Read the model definition and answer for the solid it produces. Units are mm, in the model's axes. Give positions to 0.01 mm unless a question says otherwise; leave off trailing zeros. Order: outer loops, then holes, each group sorted by start corner. A loop starts at its lowest first (then second) coordinate and runs counter-clockwise, first axis right, second up. Notation, with made-up numbers: M 50.5,14 L 54.5,14 A22 cw 54.5,40 Z; hole C -12,34 d5. An arc over 180 degrees is marked long. One line per item, written item: value.
from build123d import *

# Parameters (mm, degrees)
F3_DEPTH = 25.4


# Not quite as in the source:
# - the program builds the solid bodies; features that only make, move or delete a surface that nothing else refers to are left out


with BuildPart() as f3:
    # F2 (on Right) → F3 (new body)
    with BuildSketch(Plane.YZ):
        Polygon((62.2603967786, 39.2553694546), (-65.4462724924, 39.2553694546), (-95.9557369351, 0), (0, 0), (27.4173058569, 3.0065653846), align=None)
    extrude(amount=F3_DEPTH)


solid = f3.part
1) Consider probe 1 along Z at (x, y) = (14.75, 38.5); probe 2 along Z at (x, y) = (1.5, 30); probe 3 along Y at (x, z) = (7.25, 11). Determine where each line is inside the solid, lowest interval first.
Reported:
probe 1: z = 14.54 to 39.26
probe 2: z = 5.69 to 39.26
probe 3: y = -87.41 to 35.1
2) Find section C-C, the plane z = 18. Write down the section's boundary in (x, y), plus the area to 3 significant figures.
Reported:
outline: M 0,-81.97 L 25.4,-81.97 L 25.4,41.83 L 0,41.83 Z
area: 3,140 mm^2
3) Find section A-A, the plane x = 12.5. Write down the section's boundary in (y, z).
Reported:
outline: M -95.96,0 L 0,0 L 27.42,3.01 L 62.26,39.26 L -65.45,39.26 Z
4) Each of these flat-tipped pins is pushed along its axis until it touches: pin 1 Ø5 at (x, z) = (6.5, 6.5) entering from -Y; pin 2 Ø10 at (x, z) = (4, 19) entering from -Y. Where does it stop, or does it pass through?
Reported:
pin 1: stops at y = -92.85
pin 2: stops at y = -85.07
5) Find section B-B, the plane y = -72.5. Write down the section's boundary in (x, z), plus the area to 3 significant figures.
Reported:
outline: M 0,0 L 25.4,0 L 25.4,30.18 L 0,30.18 Z
area: 767 mm^2
